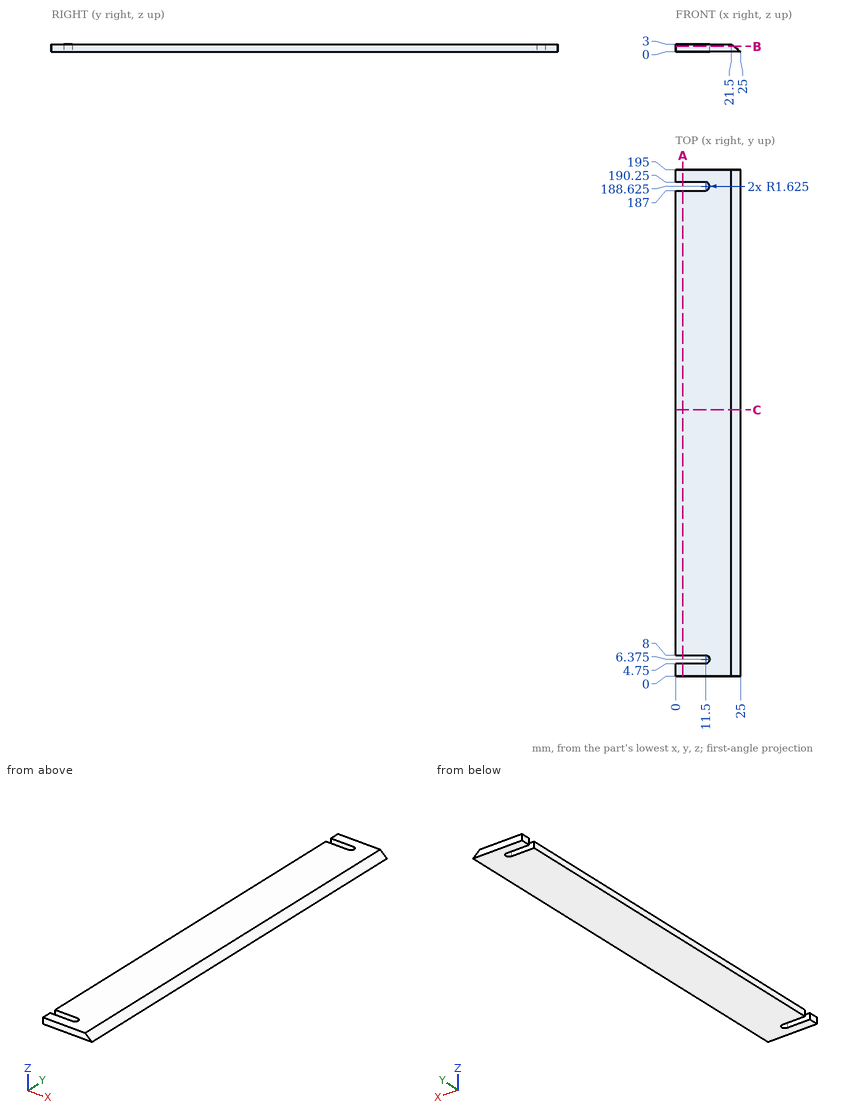
Design review of the part shown in the three views and the two pictorial views. Dimensions are in mm from the part's minimum x, y and z. Round coordinates to 2 decimals unless told otherwise and drop trailing zeros. Order: outer loops, then holes, each group sorted by start corner. A loop starts at its lowest first (then second) coordinate and runs counter-clockwise, first axis right, second up. Notation, with made-up numbers: M 5,13 L 34,13 A34 ccw 34,50 Z; hole C -35,79 d5. An arc over 180 degrees is marked long. Put each result on its own line as item: value.
Q1. Consider section B-B (z = 2.05). State the section outline as (x, y) points (3 decimals), and give its area (3 significant figures).
Reported:
outline: M 0,0 L 22.608,0 L 22.608,195 L 0,195 L 0,190.25 L 11.5,190.25 A1.625 cw 11.5,187 L 0,187 L 0,8 L 11.5,8 A1.625 cw 11.5,4.75 L 0,4.75 Z
area: 4,330 mm²
Q2. Consider section A-A (x = 2.75). State the section outline as (y, z) points.
Reported:
outline: M 0,0 L 4.75,0 L 4.75,3 L 0,3 Z; M 8,0 L 187,0 L 187,3 L 8,3 Z; M 190.25,0 L 195,0 L 195,3 L 190.25,3 Z
Q3. Insertion check: pin 1 Ø1 at (y, z) = (77.5, 0.5) entering from -X. The pin has a flat end and moves straight along its axis. Give the tip position at first contact, or say it passes through.
Reported:
pin 1: x = 0
Q4. Consider section C-C (y = 102.5). State the section outline as (x, z) points.
Reported:
outline: M 0,0 L 25,0 L 21.5,3 L 0,3 Z
Q5. To check wall thickness, follow line 1 (Y direction, x = 5.25, z = 2.05); line 2 (Y direction, x = 12.75, z = 1.1); line 3 (X direction, y = 102.5, z = 2.3). State the ranges of each line that lie inside material, in increasing order.
Reported:
line 1: 0 to 4.75, 8 to 187, 190.25 to 195
line 2: 0 to 5.34, 7.41 to 187.59, 189.66 to 195
line 3: 0 to 22.32
